Read the model definition and answer for the solid it produces. Units are mm, in the model's axes. Face numbers are marked on the shaded views. A direction names the side the tool comes from. Round coordinates to 2 decimals unless told otherwise and drop trailing zeros. Order: outer loops, then holes, each group sorted by start corner. A loop starts at its lowest first (then second) coordinate and runs counter-clockwise, first axis right, second up. Notation, with made-up numbers: (-30, 31.5) - (-12, 31.5) arc R11 ccw to (-12, 42.5) - close; hole circle Ø7 at (49.5, 27.5). An arc over 180 degrees is marked (long way). Put each result on its own line as item: value. Start each with the question number.
Q1. Find the intervals of material crossed by line 1 along Y through (x, z) = (-12.5, 1.3); line 2 along Y through (x, z) = (3, 0.25); line 3 along X through (y, z) = (-12, 0.25), in increasing order. Write a range as from..to.
Q2. Each of these flat-tipped pins is pushed along its axis until it touches: pin 1 Ø4.5 at (x, y) = (-12.5, 12.5) entering from -Z; pin 2 Ø8.5 at (y, z) = (21, -6.5) entering from -X; pin 3 Ø2 at (x, z) = (-5, 0.5) entering from +Y. Where does it stop, or does it pass through?
Q3. Section D-D on y = 15 is taken. Give the vertices of the cut face in (x, z).
Q4. Section A-A on x = -12.5 is taken. Give the vertices of the cut face in (y, z), then the cut area to 3 significant figures.
Q5. Section C-C on y = -12.5 is taken. Give the vertices of the cut face in (x, z).
Q6. Which of the six approach directions +Z, -Z, +X, -X, +Y, -Y give full straight-line access (tool end or side, diameter ignored) to the marked faces 1 and 2?
Q7. Section B-B on x = 12.5 is taken. Give the vertices of the cut face in (y, z), then the cut area to 3 significant figures.
from build123d import *

# Parameters (mm, degrees)
SKETCH2_W           = 33
SKETCH2_H           = 33
BOSS_EXTRUDE1_DEPTH = 2
BOSS_EXTRUDE2_DEPTH = 2
SKETCH4_R           = 1.5
CUT_EXTRUDE1_DEPTH  = 2
SKETCH5_R           = 2
SKETCH5_W           = 12.798144854
SKETCH5_H           = 2.519841992
CUT_EXTRUDE2_DEPTH  = 2


with BuildPart() as part:
    # Sketch2 → Boss-Extrude1 (new body)
    with BuildSketch(Plane.XY):
        Rectangle(SKETCH2_W, SKETCH2_H)
    extrude(amount=BOSS_EXTRUDE1_DEPTH)

    # Sketch3 → Boss-Extrude2 (add)
    with BuildSketch(Plane(origin=(16.5, 0, 0), x_dir=(0, 0, -1), z_dir=(1, 0, 0))):
        Polygon((3.554468931, 0.544368727), (0, -6.342288665), (0, 11.100222554), (10.205017704, 30.872082142), (17.313955565, 27.202885706), align=None)
    extrude(amount=-BOSS_EXTRUDE2_DEPTH)

    # Sketch4 → Cut-Extrude1 (cut)
    with BuildSketch(Plane(origin=(16.5, 0, 0), x_dir=(0, 0, -1), z_dir=(1, 0, 0))):
        with Locations((6.13151514, 14.258559898)):
            Circle(SKETCH4_R)
        with Locations((9.994536788, 21.743027229)):
            Circle(SKETCH4_R)
    extrude(amount=-CUT_EXTRUDE1_DEPTH, mode=Mode.SUBTRACT)

    # Sketch5 → Cut-Extrude2 (cut)
    with BuildSketch(Plane(origin=(0, 0, 0), x_dir=(-1, 0, 0), z_dir=(0, 0, -1))):
        with Locations((12.5, 12.5)):
            Circle(SKETCH5_R)
        with Locations((12.5, -12.5)):
            Circle(SKETCH5_R)
        with Locations((-12.5, -12.5)):
            Circle(SKETCH5_R)
        with Locations((0, -12.077487842)):
            Rectangle(SKETCH5_W, SKETCH5_H)
    extrude(amount=-CUT_EXTRUDE2_DEPTH, mode=Mode.SUBTRACT)


solid = part.part
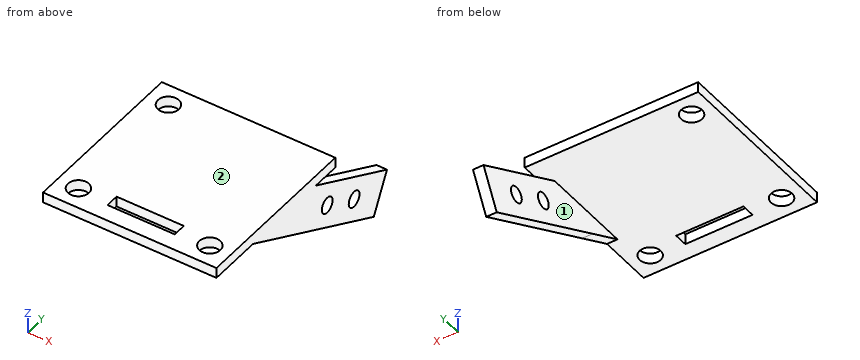
Findings:
1. line 1: -16.5..-14.5, -10.5..10.5, 14.5..16.5
1. line 2: -16.5..-13.34, -10.82..16.5
1. line 3: -16.5..-14.44, -10.56..-6.4, 6.4..10.56, 14.44..16.5
2. pin 1: z = 0
2. pin 2: x = 14.5
2. pin 3: y = 16.5
3. outline: (-16.5, 0) - (16.5, 0) - (16.5, 2) - (-16.5, 2) - close; (14.5, -11.02) - (16.5, -11.02) - (16.5, -7.44) - (14.5, -7.44) - close; (14.5, -4.83) - (16.5, -4.83) - (16.5, -2.01) - (14.5, -2.01) - close
4. outline: (-16.5, 0) - (-14.5, 0) - (-14.5, 2) - (-16.5, 2) - close; (-10.5, 0) - (10.5, 0) - (10.5, 2) - (-10.5, 2) - close; (14.5, 0) - (16.5, 0) - (16.5, 2) - (14.5, 2) - close
4. area: 50.0 mm2
5. outline: (-16.5, 0) - (-14.5, 0) - (-14.5, 2) - (-16.5, 2) - close; (-10.5, 0) - (-6.4, 0) - (-6.4, 2) - (-10.5, 2) - close; (6.4, 0) - (10.5, 0) - (10.5, 2) - (6.4, 2) - close; (14.5, 0) - (16.5, 0) - (16.5, 2) - (14.5, 2) - close
6. face 1: -Z, -X, +Y, -Y
6. face 2: +Z, +X, -X, +Y, -Y
7. outline: (-16.5, 0) - (-14.5, 0) - (-14.5, 2) - (-16.5, 2) - close; (-10.5, 0) - (16.5, 0) - (16.5, 2) - (-10.5, 2) - close
7. area: 58.0 mm2
